The listing builds one solid part. Answer for the finished solid, in the listing's coordinates (mm). Face numbers are marked on the shaded views. Coordinates: 2 decimals unless noted, no trailing zeros. Loops run counter-clockwise (first coordinate to the right, second up) from the corner with the lowest first, then second, coordinate; pieces in that order, holes last. Notation, with made-up numbers: M 57.5,25 L 76.5,25 A3 ccw 76.5,30 Z; hole C 84,75 d10. An arc over 180 degrees is marked long. Answer as a JSON object with one key per item and string values. Group by question number.
1. A cutting plane is placed at D-D on x = -10.5. Give the vertices of the cut face in (y, z).
2. A cutting plane is placed at C-C on y = -9.5. Give the vertices of the cut face in (x, z), and give its area (3 significant figures).
3. A cutting plane is placed at A-A on y = 0. Give the vertices of the cut face in (x, z), and give its area (3 significant figures).
4. Determine the mould class of the marked faces 1, 2 and 3 for opening direction X: released by +X, released by -X, zero draft, split by the parting line, or undercut.
5. Straight lines are drawn through the part: L1, parallel to Y at x = -14, z = 2.8; L2, parallel to Y at x = 4, z = 0.4. For each, find the intervals that lie inside material, in ascending order.
6. Given pin 1 (2 mm diameter, centred on y = 6, z = 1, fed in from +X); pin 2 (1.5 mm diameter, centred on x = -12.5, z = 3.5, fed in from +Y); pin 3 (1 mm diameter, centred on y = -9.5, z = 1, fed in from +X), each flat-ended and moving along its own axis, determine where each tip first touches the part or whether it passes through.
7. A cutting plane is placed at B-B on x = 12. Give the vertices of the cut face in (y, z).
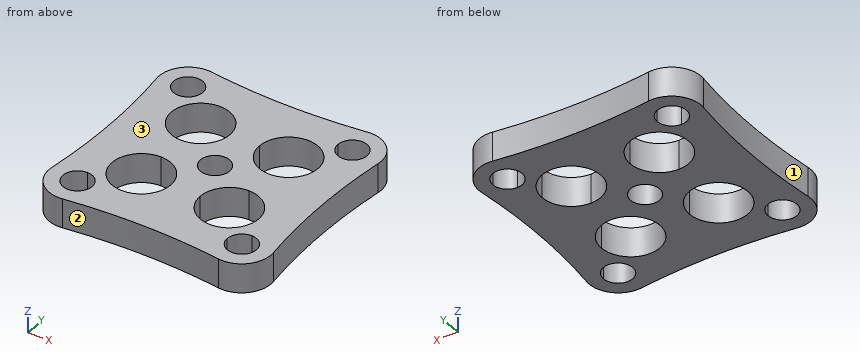
from build123d import *

# Parameters (mm, degrees)
F0_R     = 2.5
F1_DEPTH = 5
F2_R     = 5


with BuildPart() as f1:
    # F0 (on Top) → F1 (new body)
    with BuildSketch(Plane.XY):
        with BuildLine():
            ThreePointArc((-20, -20), (0, -18), (20, -20))
            ThreePointArc((20, -20), (18, 0), (20, 20))
            ThreePointArc((20, 20), (0, 18), (-20, 20))
            ThreePointArc((-20, 20), (-18, 0), (-20, -20))
        make_face()
        with BuildLine():
            ThreePointArc((16.5, 14), (15.767766953, 12.232233047), (14, 11.5))
            Line((14, 11.5), (14, -11.5))
            ThreePointArc((14, -11.5), (15.767766953, -12.232233047), (16.5, -14))
            ThreePointArc((16.5, -14), (14, -16.5), (11.5, -14))
            Line((11.5, -14), (-11.5, -14))
            ThreePointArc((-11.5, -14), (-15.767766953, -15.767766953), (-14, -11.5))
            Line((-14, -11.5), (-14, 11.5))
            ThreePointArc((-14, 11.5), (-15.767766953, 15.767766953), (-11.5, 14))
            Line((-11.5, 14), (11.5, 14))
            ThreePointArc((11.5, 14), (14, 16.5), (16.5, 14))
        make_face(mode=Mode.SUBTRACT)
        with BuildLine():
            Line((14, -11.5), (14, 11.5))
            ThreePointArc((14, 11.5), (12.232233047, 12.232233047), (11.5, 14))
            Line((11.5, 14), (-11.5, 14))
            ThreePointArc((-11.5, 14), (-12.232233047, 12.232233047), (-14, 11.5))
            Line((-14, 11.5), (-14, -11.5))
            ThreePointArc((-14, -11.5), (-12.232233047, -12.232233047), (-11.5, -14))
            Line((-11.5, -14), (11.5, -14))
            ThreePointArc((11.5, -14), (12.232233047, -12.232233047), (14, -11.5))
        make_face()
        with BuildLine():
            Line((2.5, -7.5), (-2.5, -7.5))
            ThreePointArc((-2.5, -7.5), (-11.0355339059, -11.0355339059), (-7.5, -2.5))
            Line((-7.5, -2.5), (-7.5, 2.5))
            ThreePointArc((-7.5, 2.5), (-11.0355339059, 11.0355339059), (-2.5, 7.5))
            Line((-2.5, 7.5), (2.5, 7.5))
            ThreePointArc((2.5, 7.5), (7.5, 12.5), (12.5, 7.5))
            ThreePointArc((12.5, 7.5), (11.0355339059, 3.9644660941), (7.5, 2.5))
            Line((7.5, 2.5), (7.5, -2.5))
            ThreePointArc((7.5, -2.5), (11.0355339059, -3.9644660941), (12.5, -7.5))
            ThreePointArc((12.5, -7.5), (7.5, -12.5), (2.5, -7.5))
        make_face(mode=Mode.SUBTRACT)
        with BuildLine():
            ThreePointArc((-7.5, -2.5), (-3.9644660941, -3.9644660941), (-2.5, -7.5))
            Line((-2.5, -7.5), (2.5, -7.5))
            ThreePointArc((2.5, -7.5), (3.9644660941, -3.9644660941), (7.5, -2.5))
            Line((7.5, -2.5), (7.5, 2.5))
            ThreePointArc((7.5, 2.5), (3.9644660941, 3.9644660941), (2.5, 7.5))
            Line((2.5, 7.5), (-2.5, 7.5))
            ThreePointArc((-2.5, 7.5), (-3.9644660941, 3.9644660941), (-7.5, 2.5))
            Line((-7.5, 2.5), (-7.5, -2.5))
        make_face()
        Circle(F0_R, mode=Mode.SUBTRACT)
    extrude(amount=F1_DEPTH)

    # F2
    f2_edges = [f1.edges().sort_by_distance(p)[0] for p in [
        (20, -20, 2.5),
        (-20, -20, 2.5),
        (20, 20, 2.5),
        (-20, 20, 2.5),
    ]]
    fillet(f2_edges, radius=F2_R)


solid = f1.part
From the geometry:
{
 "1": {"outline": "M -18.55,0 L -11.5,0 L -11.5,5 L -18.55,5 Z; M -3.5,0 L 3.5,0 L 3.5,5 L -3.5,5 Z; M 11.5,0 L 18.55,0 L 18.55,5 L 11.5,5 Z"},
 "2": {"outline": "M -18.45,0 L -12.08,0 L -12.08,5 L -18.45,5 Z; M -2.92,0 L 2.92,0 L 2.92,5 L -2.92,5 Z; M 12.08,0 L 18.45,0 L 18.45,5 L 12.08,5 Z", "area": "92.8 mm²"},
 "3": {"outline": "M -18,0 L -2.5,0 L -2.5,5 L -18,5 Z; M 2.5,0 L 18,0 L 18,5 L 2.5,5 Z", "area": "155 mm²"},
 "4": {"face 1": "released by -X", "face 2": "undercut", "face 3": "zero draft"},
 "5": {"L1": "y = -18.92 to -16.5, -11.5 to 11.5, 16.5 to 18.92", "L2": "y = -18.08 to -11.07, -3.93 to 3.93, 11.07 to 18.08"},
 "6": {"pin 1": "stops at x = 18.24", "pin 2": "stops at y = 18.87", "pin 3": "stops at x = 18.5"},
 "7": {"outline": "M -18.72,0 L -15.5,0 L -15.5,5 L -18.72,5 Z; M -12.5,0 L -9.68,0 L -9.68,5 L -12.5,5 Z; M -5.32,0 L 5.32,0 L 5.32,5 L -5.32,5 Z; M 9.68,0 L 12.5,0 L 12.5,5 L 9.68,5 Z; M 15.5,0 L 18.72,0 L 18.72,5 L 15.5,5 Z"}
}
